from build123d import *

# Parameters (mm, degrees)
SKETCH2_R                = 1.5
SKETCH2_R_2              = 11
SKETCH2_R_3              = 1.65
SKETCH2_R_4              = 1
BOSS_EXTRUDE1_DEPTH      = 4
M4_CLEARANCE_HOLE1_D     = 4.3
M4_CLEARANCE_HOLE1_DEPTH = 6
M4_CLEARANCE_HOLE1_TIP   = 1.291850331
M3_CLEARANCE_HOLE2_D     = 3.2
M3_CLEARANCE_HOLE2_DEPTH = 6
M3_CLEARANCE_HOLE2_TIP   = 0.96137699
M5_TAPPED_HOLE1_D        = 4.2
M5_TAPPED_HOLE1_DEPTH    = 12.4
M5_TAPPED_HOLE1_TIP      = 1.2618073
M6_CLEARANCE_HOLE1_D     = 6.4
M6_CLEARANCE_HOLE1_DEPTH = 15
M6_CLEARANCE_HOLE1_TIP   = 1.922753981
M3_TAPPED_HOLE2_D        = 2.5
M3_TAPPED_HOLE2_DEPTH    = 7.5
M3_TAPPED_HOLE2_TIP      = 0.751075774


with BuildPart() as part:
    # Sketch2 → Boss-Extrude1 (new body)
    with BuildSketch(Plane.XY):
        with BuildLine():
            Line((-140, 175), (-115.60032364, 175))
            ThreePointArc((-115.60032364, 175), (-112.064789734, 173.535533906), (-110.60032364, 170))
            Line((-110.60032364, 170), (-110.60032364, 167))
            ThreePointArc((-110.60032364, 167), (-109.135857546, 163.464466094), (-105.60032364, 162))
            Line((-105.60032364, 162), (105.60032364, 162))
            ThreePointArc((105.60032364, 162), (109.135857546, 163.464466094), (110.60032364, 167))
            Line((110.60032364, 167), (110.60032364, 170))
            ThreePointArc((110.60032364, 170), (112.064789734, 173.535533906), (115.60032364, 175))
            Line((115.60032364, 175), (140, 175))
            ThreePointArc((140, 175), (143.535533906, 173.535533906), (145, 170))
            Line((145, 170), (145, 57))
            ThreePointArc((145, 57), (144.414213562, 55.585786438), (143, 55))
            Line((143, 55), (132, 55))
            ThreePointArc((132, 55), (130.585786438, 54.414213562), (130, 53))
            Line((130, 53), (130, -3))
            ThreePointArc((130, -3), (130.585786438, -4.414213562), (132, -5))
            Line((132, -5), (143, -5))
            ThreePointArc((143, -5), (144.414213562, -5.585786438), (145, -7))
            Line((145, -7), (145, -120))
            ThreePointArc((145, -120), (143.535533906, -123.535533906), (140, -125))
            Line((140, -125), (115.60032364, -125))
            ThreePointArc((115.60032364, -125), (112.064789734, -123.535533906), (110.60032364, -120))
            Line((110.60032364, -120), (110.60032364, -117))
            ThreePointArc((110.60032364, -117), (109.135857546, -113.464466094), (105.60032364, -112))
            Line((105.60032364, -112), (-105.60032364, -112))
            ThreePointArc((-105.60032364, -112), (-109.135857546, -113.464466094), (-110.60032364, -117))
            Line((-110.60032364, -117), (-110.60032364, -120))
            ThreePointArc((-110.60032364, -120), (-112.064789734, -123.535533906), (-115.60032364, -125))
            Line((-115.60032364, -125), (-140, -125))
            ThreePointArc((-140, -125), (-143.535533906, -123.535533906), (-145, -120))
            Line((-145, -120), (-145, -7))
            ThreePointArc((-145, -7), (-144.414213562, -5.585786438), (-143, -5))
            Line((-143, -5), (-132, -5))
            ThreePointArc((-132, -5), (-130.585786438, -4.414213562), (-130, -3))
            Line((-130, -3), (-130, 53))
            ThreePointArc((-130, 53), (-130.585786438, 54.414213562), (-132, 55))
            Line((-132, 55), (-143, 55))
            ThreePointArc((-143, 55), (-144.414213562, 55.585786438), (-145, 57))
            Line((-145, 57), (-145, 170))
            ThreePointArc((-145, 170), (-143.535533906, 173.535533906), (-140, 175))
        make_face()
        with Locations((-132.473303105, 168.56037538)):
            Circle(SKETCH2_R, mode=Mode.SUBTRACT)
        with Locations((-132.473303105, 139.890769728)):
            Circle(SKETCH2_R, mode=Mode.SUBTRACT)
        with Locations((132.473303105, 168.56037538)):
            Circle(SKETCH2_R, mode=Mode.SUBTRACT)
        with Locations((132.473303105, 139.890769728)):
            Circle(SKETCH2_R, mode=Mode.SUBTRACT)
        with Locations((132.473303105, 154.225572554)):
            Circle(SKETCH2_R_2, mode=Mode.SUBTRACT)
        with Locations((-132.473303105, 154.225572554)):
            Circle(SKETCH2_R_2, mode=Mode.SUBTRACT)
        with Locations((121.59774802, -0.5)):
            Circle(SKETCH2_R_3, mode=Mode.SUBTRACT)
        with Locations((121.59774802, 50.5)):
            Circle(SKETCH2_R_3, mode=Mode.SUBTRACT)
        with Locations((-121.59774802, -0.5)):
            Circle(SKETCH2_R_3, mode=Mode.SUBTRACT)
        with Locations((-121.59774802, 50.5)):
            Circle(SKETCH2_R_3, mode=Mode.SUBTRACT)
        with Locations((-29, 10)):
            Circle(SKETCH2_R, mode=Mode.SUBTRACT)
        with Locations((-29, 40)):
            Circle(SKETCH2_R, mode=Mode.SUBTRACT)
        with Locations((-53, 40)):
            Circle(SKETCH2_R, mode=Mode.SUBTRACT)
        with Locations((-53, 10)):
            Circle(SKETCH2_R, mode=Mode.SUBTRACT)
        with Locations((53, 10)):
            Circle(SKETCH2_R, mode=Mode.SUBTRACT)
        with Locations((29, 10)):
            Circle(SKETCH2_R, mode=Mode.SUBTRACT)
        with Locations((29, 40)):
            Circle(SKETCH2_R, mode=Mode.SUBTRACT)
        with Locations((53, 40)):
            Circle(SKETCH2_R, mode=Mode.SUBTRACT)
        with Locations((132.473303105, -118.56037538)):
            Circle(SKETCH2_R, mode=Mode.SUBTRACT)
        with Locations((132.473303105, -89.890769728)):
            Circle(SKETCH2_R, mode=Mode.SUBTRACT)
        with Locations((132.473303105, -104.225572554)):
            Circle(SKETCH2_R_2, mode=Mode.SUBTRACT)
        with Locations((-132.473303105, -104.225572554)):
            Circle(SKETCH2_R_2, mode=Mode.SUBTRACT)
        with Locations((-132.473303105, -89.890769728)):
            Circle(SKETCH2_R, mode=Mode.SUBTRACT)
        with Locations((-132.473303105, -118.56037538)):
            Circle(SKETCH2_R, mode=Mode.SUBTRACT)
        with Locations((130, 75)):
            Circle(SKETCH2_R, mode=Mode.SUBTRACT)
        with Locations((41.5, 95.575)):
            Circle(SKETCH2_R_4, mode=Mode.SUBTRACT)
        with Locations((41.5, 80.575)):
            Circle(SKETCH2_R_4, mode=Mode.SUBTRACT)
        with Locations((-20, 80.575)):
            Circle(SKETCH2_R_4, mode=Mode.SUBTRACT)
        with Locations((-20, 95.575)):
            Circle(SKETCH2_R_4, mode=Mode.SUBTRACT)
        with Locations((-20, -45.575)):
            Circle(SKETCH2_R_4, mode=Mode.SUBTRACT)
        with Locations((-20, -30.575)):
            Circle(SKETCH2_R_4, mode=Mode.SUBTRACT)
        with Locations((41.5, -30.575)):
            Circle(SKETCH2_R_4, mode=Mode.SUBTRACT)
        with Locations((41.5, -45.575)):
            Circle(SKETCH2_R_4, mode=Mode.SUBTRACT)
        with Locations((130, -25)):
            Circle(SKETCH2_R, mode=Mode.SUBTRACT)
        with Locations((-130, 75)):
            Circle(SKETCH2_R, mode=Mode.SUBTRACT)
        with Locations((-130, -25)):
            Circle(SKETCH2_R, mode=Mode.SUBTRACT)
        with Locations((87.5, 147.175)):
            Circle(SKETCH2_R_4, mode=Mode.SUBTRACT)
        with Locations((37.5, 147.175)):
            Circle(SKETCH2_R_4, mode=Mode.SUBTRACT)
        with Locations((-37.5, 147.175)):
            Circle(SKETCH2_R_4, mode=Mode.SUBTRACT)
        with Locations((-87.5, 147.175)):
            Circle(SKETCH2_R_4, mode=Mode.SUBTRACT)
        with Locations((-87.5, -97.175)):
            Circle(SKETCH2_R_4, mode=Mode.SUBTRACT)
        with Locations((-37.5, -97.175)):
            Circle(SKETCH2_R_4, mode=Mode.SUBTRACT)
        with Locations((37.5, -97.175)):
            Circle(SKETCH2_R_4, mode=Mode.SUBTRACT)
        with Locations((87.5, -97.175)):
            Circle(SKETCH2_R_4, mode=Mode.SUBTRACT)
        with BuildLine():
            Line((-66, 62.171403079), (-111.59774802, 62.171403079))
            ThreePointArc((-111.59774802, 62.171403079), (-114.426175145, 60.999830204), (-115.59774802, 58.171403079))
            Line((-115.59774802, 58.171403079), (-115.59774802, -8.171403079))
            ThreePointArc((-115.59774802, -8.171403079), (-114.426175145, -10.999830204), (-111.59774802, -12.171403079))
            Line((-111.59774802, -12.171403079), (-66, -12.171403079))
            ThreePointArc((-66, -12.171403079), (-63.171572875, -10.999830204), (-62, -8.171403079))
            Line((-62, -8.171403079), (-62, 58.171403079))
            ThreePointArc((-62, 58.171403079), (-63.171572875, 60.999830204), (-66, 62.171403079))
        make_face(mode=Mode.SUBTRACT)
        with BuildLine():
            Line((66, 62.171403079), (111.59774802, 62.171403079))
            ThreePointArc((111.59774802, 62.171403079), (114.426175145, 60.999830204), (115.59774802, 58.171403079))
            Line((115.59774802, 58.171403079), (115.59774802, -8.171403079))
            ThreePointArc((115.59774802, -8.171403079), (114.426175145, -10.999830204), (111.59774802, -12.171403079))
            Line((111.59774802, -12.171403079), (66, -12.171403079))
            ThreePointArc((66, -12.171403079), (63.171572875, -10.999830204), (62, -8.171403079))
            Line((62, -8.171403079), (62, 58.171403079))
            ThreePointArc((62, 58.171403079), (63.171572875, 60.999830204), (66, 62.171403079))
        make_face(mode=Mode.SUBTRACT)
    extrude(amount=BOSS_EXTRUDE1_DEPTH)

    # M4 Clearance Hole1
    with Locations(Plane(origin=(-53, 40, 4), x_dir=(1, 0, 0), z_dir=(0, 0, 1))):
        with Locations((0, 0), (24, 0), (24, -30), (0, -30), (82, 0), (106, 0), (106, -30), (82, -30)):
            Hole(M4_CLEARANCE_HOLE1_D / 2, depth=M4_CLEARANCE_HOLE1_DEPTH)
            with Locations((0, 0, -(M4_CLEARANCE_HOLE1_DEPTH + M4_CLEARANCE_HOLE1_TIP / 2))):  # 118° drill point
                Cone(0, M4_CLEARANCE_HOLE1_D / 2, M4_CLEARANCE_HOLE1_TIP, mode=Mode.SUBTRACT)

    # M3 Clearance Hole2
    with Locations(Plane(origin=(-132.473303105, 168.56037538, 4), x_dir=(1, 0, 0), z_dir=(0, 0, 1))):
        with Locations((0, 0), (0, -28.669605652), (264.94660621, -28.669605652), (264.94660621, 0), (173.973303105, -87.98537538), (173.973303105, -72.98537538), (112.473303105, -72.98537538), (112.473303105, -87.98537538), (173.973303105, -199.13537538), (173.973303105, -214.13537538), (112.473303105, -214.13537538), (112.473303105, -199.13537538), (264.94660621, -258.451145108), (264.94660621, -287.12075076), (0, -287.12075076), (0, -258.451145108)):
            Hole(M3_CLEARANCE_HOLE2_D / 2, depth=M3_CLEARANCE_HOLE2_DEPTH)
            with Locations((0, 0, -(M3_CLEARANCE_HOLE2_DEPTH + M3_CLEARANCE_HOLE2_TIP / 2))):  # 118° drill point
                Cone(0, M3_CLEARANCE_HOLE2_D / 2, M3_CLEARANCE_HOLE2_TIP, mode=Mode.SUBTRACT)

    # M5 Tapped Hole1
    with Locations(Plane(origin=(-121.59774802, 50.5, 4), x_dir=(1, 0, 0), z_dir=(0, 0, 1))):
        with Locations((0, 0), (0, -51), (243.19549604, -51), (243.19549604, 0)):
            Hole(M5_TAPPED_HOLE1_D / 2, depth=M5_TAPPED_HOLE1_DEPTH)
            with Locations((0, 0, -(M5_TAPPED_HOLE1_DEPTH + M5_TAPPED_HOLE1_TIP / 2))):  # 118° drill point
                Cone(0, M5_TAPPED_HOLE1_D / 2, M5_TAPPED_HOLE1_TIP, mode=Mode.SUBTRACT)

    # M6 Clearance Hole1
    with Locations(Plane(origin=(-130, 75, 4), x_dir=(1, 0, 0), z_dir=(0, 0, 1))):
        with Locations((0, 0), (260, 0), (260, -100), (0, -100)):
            Hole(M6_CLEARANCE_HOLE1_D / 2, depth=M6_CLEARANCE_HOLE1_DEPTH)
            with Locations((0, 0, -(M6_CLEARANCE_HOLE1_DEPTH + M6_CLEARANCE_HOLE1_TIP / 2))):  # 118° drill point
                Cone(0, M6_CLEARANCE_HOLE1_D / 2, M6_CLEARANCE_HOLE1_TIP, mode=Mode.SUBTRACT)

    # M3 Tapped Hole2
    with Locations(Plane(origin=(-87.5, 147.175, 4), x_dir=(1, 0, 0), z_dir=(0, 0, 1))):
        with Locations((0, 0), (50, 0), (125, 0), (175, 0), (175, -244.35), (125, -244.35), (50, -244.35), (0, -244.35)):
            Hole(M3_TAPPED_HOLE2_D / 2, depth=M3_TAPPED_HOLE2_DEPTH)
            with Locations((0, 0, -(M3_TAPPED_HOLE2_DEPTH + M3_TAPPED_HOLE2_TIP / 2))):  # 118° drill point
                Cone(0, M3_TAPPED_HOLE2_D / 2, M3_TAPPED_HOLE2_TIP, mode=Mode.SUBTRACT)


solid = part.part
Model file for the job. Use its own axes, mm. Give positions to 0.01 mm unless a question says otherwise; leave off trailing zeros. Loops run counter-clockwise (first coordinate to the right, second up) from the corner with the lowest first, then second, coordinate; pieces in that order, holes last.
Item 1: Mould opens along Y. For faces 1 (the face through (2, 27, 4)), 2 (the face through (-133.052, -24.039, 1.972)) say: +Y half, -Y half, draft (parallel to the pull), parting line (faces both ways), or undercut.
Check values:
face 1: draft
face 2: undercut
Item 2: Drop flat-ended pins along their axis: P1, Ø5, axis at x = -121.6, y = -0.5, coming from the -Z side; P2, Ø2.5, axis at x = -53, y = 10, coming from the -Z side; P3, Ø1.2, axis at y = 26, z = 2.5, coming from the -X side; P4, Ø1.2, axis at x = 90.5, z = 1, coming from the -Y side. Give the stop position or say it passes through.
Check values:
P1: stops at z = 0
P2: passes through
P3: stops at x = -130
P4: stops at y = -112
Item 3: Slice it at B-B (y = 17.5). Write the cut outline in (x, z).
Check values:
outline: (-130, 0) - (-115.6, 0) - (-115.6, 4) - (-130, 4) - close; (-62, 0) - (62, 0) - (62, 4) - (-62, 4) - close; (115.6, 0) - (130, 0) - (130, 4) - (115.6, 4) - close
Item 4: Slice it at A-A (x = -69.5). Write the cut outline in (y, z).
Check values:
outline: (-112, 0) - (-12.17, 0) - (-12.17, 4) - (-112, 4) - close; (62.17, 0) - (162, 0) - (162, 4) - (62.17, 4) - close
Item 5: Drill centre lines: line 1 along Y through (x, z) = (29, 2.9); line 2 along X through (y, z) = (19, 1.35); line 3 along X through (y, z) = (-90, 1.9). Where is each one in solid material? Low to high.
Check values:
line 1: y = -112 to 7.85, 12.15 to 37.85, 42.15 to 162
line 2: x = -130 to -115.6, -62 to 62, 115.6 to 130
line 3: x = -145 to -134.07, -130.88 to 130.88, 134.07 to 145
Item 6: Slice it at D-D (x = 0.5). Write the cut outline in (y, z).
Check values:
outline: (-112, 0) - (162, 0) - (162, 4) - (-112, 4) - close
Item 7: Slice it at C-C (z = 1.05). Give the number of separate pieces and of enclosed holes in the cut face, plus the area to 3 significant figures.
Check values:
separate pieces: 1
enclosed holes: 46
area: 69,500 mm2
